Autodesk Inventor part; units mm, degrees
ref_plane "YZ Plane" through (0, 0, 0) normal (1, 0, 0) x (0, 1, 0)
ref_plane "XZ Plane" through (0, 0, 0) normal (0, 1, 0) x (-1, 0, 0)
ref_plane "XY Plane" through (0, 0, 0) normal (0, 0, 1) x (1, 0, 0)
sketch "Эскиз1" plane through (0, 0, 0) normal (0, 0, 1) x (1, 0, 0)
  circle A0 centre (5.6, 16) radius 0.52
  circle A1 centre (5.6, 16) radius 0.8
  line L0 (7.2, 14.675) -> (7.2, 16)
  line L1 (0, 31) -> (10, 31)
  line L2 (10, 31) -> (10, 29.5)
  line L3 (10, 29.5) -> (2, 29.5)
  line L4 (0, 0) -> (9.5856, 0)
  line L5 (0, 31) -> (0, 16)
  line L6 (0, 16) -> (2, 15.5)
  line L7 (2, 15.5) -> (5.6, 14)
  line L8 (5.6, 14) -> (7.2, 14.675)
  line L9 (5.6, 14) -> (0, 14) construction
  line L10 (0, 37.2) -> (0, -6.2)
  line L11 (-2, 0) -> (12, 0)
  line L12 (4.8, 16) -> (2, 16.7)
  line L13 (2, 16.7) -> (2, 29.5)
  line L14 (7.2, 16) -> (6.4, 16)
  dimension "d0" = 62
  dimension "d1" = 29.35
  dimension "d2" = 1.5
  dimension "d3" = 1.04
  dimension "d4" = 1.6
  dimension "d5" = 28
  dimension "d6" = 31
  dimension "d7" = 32
  dimension "d8" = 5.6
  dimension "d9" = 7.2
  dimension "d10" = 10
  dimension "d12" = 2
revolve "Базовый элемент" add sketch "Эскиз1" angle 360 about axis through (0, 0, 0) along (1, 0, 0) contours L14 L0 L8 L7 L6 L5 L1 L2 L3 L13 L12 A1
revolve "Пружинные1" add sketch "Эскиз1" angle 360 about axis through (0, 0, 0) along (1, 0, 0) contours A0 | A1
fillet "Сопряжение1" radius 0.4 3 edges at (10, -31, 0) (2, -29.5, 0) (0, -31, 0)
equation "\"d3\" = SPDI"
equation "\"d4\" = SPDA"
equation "\"d8\" = SPDST"
equation "\"d9\" = SDI"
equation "\"d12\" = SD"
equation "\"d11\" = RR"
equation "\"SD2\" = 62"
equation "\"SWDT\" = 8"
equation "\"RR\" = 0.4"
equation "\"SD\" = 2"
equation "\"NND\" = 42"
equation "\"SPDA\" = 1.6"
equation "\"SPDI\" = 1.04"
equation "\"TKDM\" = 46"
equation "\"HLDM\" = 46.8"
equation "\"ABDM\" = 44"
equation "\"SDI\" = 7.2"
equation "\"SPDST\" = 5.6"
equation "\"LAB\" = 0.4"
properties part number "Манжет 1-42x62x8 ГОСТ 8752-79" material "Резина"
Verification items for the finished model (mm, model axes). A direction names the side the tool comes from. Round coordinates to 2 decimals unless told otherwise and drop trailing zeros. Order: outer loops, then holes, each group sorted by start corner. A loop starts at its lowest first (then second) coordinate and runs counter-clockwise, first axis right, second up.
1. Access from +Z, -Z, +X, -X, +Y, -Y to the whole of each face (thin tool, end or side, straight path). Record for faces 1 (the flat face through (10, -16, 25)), 2 (the conical face through (4.625, -3.478, 15.662)), 3 (the flat face through (7.2, 14, -5)).
Final values:
face 1: +Z, -Z, +X, +Y, -Y
face 2: none
face 3: +X
2. Section check C-C on x = 8.75. Record the cut outline in (y, z), then the cut area to 3 significant figures.
Final values:
outline: circle Ø62 at (0, 0); hole circle Ø59 at (0, 0)
area: 285 mm2
3. Go/stop test with flat-tipped pins: P1, Ø6, axis at x = 2, y = -3.5, coming from the +Z side; P2, Ø6, axis at x = 7, z = 18.5, coming from the +Y side; P3, Ø5, axis at x = 2.5, z = 7, coming from the +Y side. Record where each tip stops, or that it passes through.
Final values:
P1: stops at z = 31
P2: stops at y = 26.85
P3: stops at y = 30.67
4. Thickness scan on L1, parallel to Z at x = 6.75, y = 0; L2, parallel to Z at x = 7.75, y = 0.5; L3, parallel to Z at x = 2.25, y = -4. Record the ranges inside material, lowest first.
Final values:
L1: z = -31 to -29.5, -16 to -14.49, 14.49 to 16, 29.5 to 31
L2: z = -31 to -29.5, 29.5 to 31
L3: z = -30.74 to -29.2, -16.15 to -14.87, 14.87 to 16.15, 29.2 to 30.74
5. Release check for a two-part mould opening along Y. For faces 4 (the conical face through (5.375, 6.503, 12.504)), 5 (the cylindrical face through (6.79, -3.47, 15.62)), 6 (the flat face through (0, 13, -13)), 7 (the cylindrical face through (5.064, -4.036, 30.736)) record: +Y half, -Y half, draft (parallel to the pull), parting line (faces both ways), or undercut.
Final values:
face 4: undercut
face 5: undercut
face 6: draft
face 7: parting line
6. Section check D-D on x = 3.75. Record the cut outline in (y, z) (1 decimal), then the cut area to 3 significant figures.
Final values:
outline: circle Ø62 at (0, 0); circle Ø32.5 at (0, 0); hole circle Ø59 at (0, 0); hole circle Ø29.5 at (0, 0)
area: 431 mm2
